CAD build for the part. Positions are in the model's coordinates, mm. A direction names the side the tool comes from. Round coordinates to 2 decimals unless told otherwise and drop trailing zeros. Loops run counter-clockwise (first coordinate to the right, second up) from the corner with the lowest first, then second, coordinate; pieces in that order, holes last.
from build123d import *

# Parameters (mm, degrees)
ESQUISSE1_R             = 8.5
BOSS_EXTRU_1_DEPTH      = 2
BOSS_EXTRU_2_DEPTH      = 10.5
ESQUISSE3_R             = 5.5
BOSS_EXTRU_3_DEPTH      = 1
ESQUISSE4_R             = 6.35
BOSS_EXTRU_4_DEPTH      = 1.5
ESQUISSE5_R             = 2
ENL_V_MAT_EXTRU_1_DEPTH = 20.222382787


with BuildPart() as part:
    # Esquisse1 → Boss.-Extru.1 (new body)
    with BuildSketch(Plane.XY):
        Circle(ESQUISSE1_R)
    extrude(amount=BOSS_EXTRU_1_DEPTH)

    # Esquisse2 → Boss.-Extru.2 (add)
    with BuildSketch(Plane.XY.offset(2)):
        Polygon((6.35, -3.666174209), (6.35, 3.666174209), (0, 7.332348419), (-6.35, 3.666174209), (-6.35, -3.666174209), (0, -7.332348419), align=None)
    extrude(amount=BOSS_EXTRU_2_DEPTH)

    # Esquisse3 → Boss.-Extru.3 (add)
    with BuildSketch(Plane.XY.offset(12.5)):
        Circle(ESQUISSE3_R)
    extrude(amount=BOSS_EXTRU_3_DEPTH)

    # Esquisse4 → Boss.-Extru.4 (add)
    with BuildSketch(Plane.XY.offset(13.5)):
        Circle(ESQUISSE4_R)
    extrude(amount=BOSS_EXTRU_4_DEPTH)

    # Esquisse5 → Enlèv. mat.-Extru.1 (cut, through all)
    with BuildSketch(Plane.XY.offset(15)):
        Circle(ESQUISSE5_R)
    extrude(amount=-ENL_V_MAT_EXTRU_1_DEPTH, mode=Mode.SUBTRACT)


solid = part.part
Item 1: Wall check: L1, parallel to Z at x = 6, y = 1.5; L2, parallel to X at y = 2.75, z = 12.25; L3, parallel to Z at x = 7.5, y = -1. Give the ranges that are in metal, low to high.
Verdict:
L1: z = 0 to 12.5, 13.5 to 15
L2: x = -6.35 to 6.35
L3: z = 0 to 2
Item 2: 3-axis set-ups, long thin cutter, end or side, ignore diameter. For faces 1 (the flat face through (-3.219, -5.474, 7.176)), 2 (the flat face through (6.35, 0, 7)), 3 (the flat face through (-1.9, -5.4, 12.5)): which of +Z, -Z, +X, -X, +Y, -Y reach the whole face in a straight line?
Verdict:
face 1: +Z, -X, -Y
face 2: +Z, +X, +Y, -Y
face 3: none
Item 3: Mould opens along Z. For faces 4 (the flat face through (2, -2, 0)), 5 (the cylindrical face through (-1.19, -5.37, 12.99)), 6 (the flat face through (-2, 2, 15)), 7 (the cylindrical face through (4.57, 7.167, 0.986)) say: released by +Z, released by -Z, zero draft, split by the parting line, or undercut.
Verdict:
face 4: released by -Z
face 5: undercut
face 6: released by +Z
face 7: zero draft
Item 4: Cut at B-B (y = 0). List the corners of the cut face in (x, z).
Verdict:
outline: (-8.5, 0) - (-2, 0) - (-2, 15) - (-6.35, 15) - (-6.35, 13.5) - (-5.5, 13.5) - (-5.5, 12.5) - (-6.35, 12.5) - (-6.35, 2) - (-8.5, 2) - close; (2, 0) - (8.5, 0) - (8.5, 2) - (6.35, 2) - (6.35, 12.5) - (5.5, 12.5) - (5.5, 13.5) - (6.35, 13.5) - (6.35, 15) - (2, 15) - close
Item 5: Flat gauge pins, fed straight in: P1, Ø2, axis at y = -1, z = 5.5, coming from the +X side; P2, Ø1.5, axis at x = 6, z = 2, coming from the -Y side; P3, Ø2, axis at y = -0.5, z = 4.5, coming from the -X side. Where does each tip first touch, or does it go through?
Verdict:
P1: stops at x = 6.35
P2: stops at y = -6.68
P3: stops at x = -6.35
Item 6: Cut at D-D (y = -1.75). List the corners of the cut face in (x, z).
Verdict:
outline: (-8.32, 0) - (-0.97, 0) - (-0.97, 15) - (-6.1, 15) - (-6.1, 13.5) - (-5.21, 13.5) - (-5.21, 12.5) - (-6.35, 12.5) - (-6.35, 2) - (-8.32, 2) - close; (0.97, 0) - (8.32, 0) - (8.32, 2) - (6.35, 2) - (6.35, 12.5) - (5.21, 12.5) - (5.21, 13.5) - (6.1, 13.5) - (6.1, 15) - (0.97, 15) - close
Item 7: Cut at A-A (z = 6.75). List the corners of the cut face in (x, y).
Verdict:
outline: (-6.35, -3.67) - (0, -7.33) - (6.35, -3.67) - (6.35, 3.67) - (0, 7.33) - (-6.35, 3.67) - close; hole circle Ø4 at (0, 0)
Item 8: Cut at C-C (x = 2.5). List the corners of the cut face in (y, z).
Verdict:
outline: (-8.12, 0) - (8.12, 0) - (8.12, 2) - (5.89, 2) - (5.89, 12.5) - (4.9, 12.5) - (4.9, 13.5) - (5.84, 13.5) - (5.84, 15) - (-5.84, 15) - (-5.84, 13.5) - (-4.9, 13.5) - (-4.9, 12.5) - (-5.89, 12.5) - (-5.89, 2) - (-8.12, 2) - close
